```python
from build123d import *

# Parameters (mm, degrees)
SKETCH_1_W          = 51
SKETCH_1_H          = 95
EXTRUDE_1_DEPTH     = 22
SKETCH_2_R          = 1
CUT_EXTRUDE_1_DEPTH = 51


with BuildPart() as part:
    # 草图1 → 凸台-拉伸1 (new body)
    with BuildSketch(Plane(origin=(0, 0, 0), x_dir=(1, 0, 0), z_dir=(0, 1, 0))):
        Rectangle(SKETCH_1_W, SKETCH_1_H)
    extrude(amount=EXTRUDE_1_DEPTH)

    # 草图2 → 切除-拉伸1 (cut)
    with BuildSketch(Plane(origin=(25.5, 0, 0), x_dir=(0, 0, -1), z_dir=(1, 0, 0))):
        with Locations((-39.5, 11)):
            Circle(SKETCH_2_R)
    cut_extrude_1 = extrude(amount=-CUT_EXTRUDE_1_DEPTH, mode=Mode.SUBTRACT)

    # 镜向1: 切除-拉伸1 across plane
    add(cut_extrude_1.mirror(Plane.XY), mode=Mode.SUBTRACT)


solid = part.part
```
Geometry check sheet. Reference: the model listing, model coordinates, mm. Give positions to 0.01 mm unless a question says otherwise; leave off trailing zeros. Loops run counter-clockwise (first coordinate to the right, second up) from the corner with the lowest first, then second, coordinate; pieces in that order, holes last. Notation, with made-up numbers: M -12.5,4.5 L 32.5,4.5 A18 cw 32.5,37.5 Z; hole C -26.75,79 d4. An arc over 180 degrees is marked long. Write item = value, one per line.
(1) Release check for a two-part mould opening along Y. For faces 1 (the face through (0.357, 11.3, 38.546)), 2 (the face through (0, 0, -1)), 3 (the face through (0, 11, -47.5)) record: released by +Y, released by -Y, zero draft, split by the parting line, or undercut.
Answer below:
face_1 = undercut
face_2 = released by -Y
face_3 = zero draft
(2) Material ranges on line 1 (Y direction, x = 2, z = 39.5); line 2 (Z direction, x = -14.5, y = 11.75), recorded low to high. Write a range as [from, to].
Answer below:
line_1 = [0, 10], [12, 22]
line_2 = [-47.5, -40.16], [-38.84, 38.84], [40.16, 47.5]
(3) Sectioned sample at A-A, the plane z = -39.5. Record the cut outline in (x, y).
Answer below:
outline = M -25.5,0 L 25.5,0 L 25.5,10 L -25.5,10 Z; M -25.5,12 L 25.5,12 L 25.5,22 L -25.5,22 Z
